```python
from build123d import *

# Parameters (mm, degrees)
SKETCH1_W           = 19.2
SKETCH1_H           = 19.2
SKETCH1_W_2         = 13.2
SKETCH1_H_2         = 13.2
BOSS_EXTRUDE1_DEPTH = 30
CUT_EXTRUDE1_DEPTH  = 30
BOSS_EXTRUDE2_DEPTH = 19.2
SKETCH4_R           = 1.28
CUT_EXTRUDE2_DEPTH  = 30
SKETCH5_R           = 2.18
CUT_EXTRUDE3_DEPTH  = 1
SKETCH6_W           = 10
SKETCH6_H           = 2.5
CUT_EXTRUDE4_DEPTH  = 3
BOSS_EXTRUDE3_DEPTH = 1
SKETCH8_W           = 4
SKETCH8_H           = 3
CUT_EXTRUDE5_DEPTH  = 4
FILLET1_R           = 0.5
FILLET2_R           = 0.5


with BuildPart() as part:
    # Sketch1 → Boss-Extrude1 (new body)
    with BuildSketch(Plane(origin=(0, 0, 0), x_dir=(1, 0, 0), z_dir=(0, 1, 0))):
        Rectangle(SKETCH1_W, SKETCH1_H)
        Rectangle(SKETCH1_W_2, SKETCH1_H_2, mode=Mode.SUBTRACT)
    extrude(amount=-BOSS_EXTRUDE1_DEPTH)

    # Sketch2 → Cut-Extrude1 (cut)
    with BuildSketch(Plane.XY.offset(9.6)):
        Polygon((-9.6, -30), (-9.6, -10), (25.041016151, -30), align=None)
    extrude(amount=-CUT_EXTRUDE1_DEPTH, mode=Mode.SUBTRACT)

    # Sketch3 → Boss-Extrude2 (add)
    with BuildSketch(Plane.XY.offset(9.6)):
        Polygon((-9.6, -10), (-9.6, -12.886751346), (15.662177826, -27.471876514), (15.662177826, -24.585125168), align=None)
    extrude(amount=-BOSS_EXTRUDE2_DEPTH)

    # Sketch4 → Cut-Extrude2 (cut)
    with BuildSketch(Plane(origin=(-6.730127019, -11.656921938, 0), x_dir=(0.866025404, -0.5, 0), z_dir=(0.5, 0.866025404, 0))):
        with Locations(Location((22.558741962, 0, 0), (0, 0, 180))):  # turned: the seam where the file's is
            Circle(SKETCH4_R)
    extrude(amount=-CUT_EXTRUDE2_DEPTH, mode=Mode.SUBTRACT)

    # Sketch5 → Cut-Extrude3 (cut)
    with BuildSketch(Plane(origin=(-6.730127019, -11.656921938, 0), x_dir=(0.866025404, -0.5, 0), z_dir=(0.5, 0.866025404, 0))):
        with Locations(Location((22.558741962, 0, 0), (0, 0, 180))):  # turned: the seam where the file's is
            Circle(SKETCH5_R)
    extrude(amount=-CUT_EXTRUDE3_DEPTH, mode=Mode.SUBTRACT)

    # Sketch6 → Cut-Extrude4 (cut)
    with BuildSketch(Plane(origin=(9.6, 0, 0), x_dir=(0, 0, -1), z_dir=(1, 0, 0))):
        with Locations((0, -15)):
            Rectangle(SKETCH6_W, SKETCH6_H)
    extrude(amount=-CUT_EXTRUDE4_DEPTH, mode=Mode.SUBTRACT)

    # Sketch7 → Boss-Extrude3 (add, symmetric)
    with BuildSketch(Plane.XY):
        Polygon((-6.6, -4.2), (-6.6, -1.2), (-4.6, -1.2), align=None)
        Polygon((6.6, -1.2), (4.6, -1.2), (6.6, -4.2), align=None)
    extrude(amount=BOSS_EXTRUDE3_DEPTH, both=True)

    # Sketch8 → Cut-Extrude5 (cut)
    with BuildSketch(Plane(origin=(0, 0, 0), x_dir=(1, 0, 0), z_dir=(0, 1, 0))):
        with Locations((0, 8.1)):
            Rectangle(SKETCH8_W, SKETCH8_H)
        with Locations((0, -8.1)):
            Rectangle(SKETCH8_W, SKETCH8_H)
    extrude(amount=-CUT_EXTRUDE5_DEPTH, mode=Mode.SUBTRACT)

    # Fillet1
    fillet1_edges = [part.edges().sort_by_distance(p)[0] for p in [
        (-6.6, -1.2, 0),
        (6.6, -1.2, 0),
    ]]
    fillet(fillet1_edges, radius=FILLET1_R)

    # Fillet2
    fillet2_edges = [part.edges().sort_by_distance(p)[0] for p in [
        (-5.8, 0, -9.6),
        (9.6, 0, 0),
        (-5.8, 0, 9.6),
        (5.8, 0, 9.6),
        (5.8, 0, -9.6),
        (-9.6, -6.443375673, 9.6),
        (9.6, -10.542562584, 9.6),
        (9.6, -10.542562584, -9.6),
        (-9.6, -6.443375673, -9.6),
        (9.6, -21.085125168, 0),
        (15.662177826, -24.585125168, 0),
        (12.631088913, -22.835125168, 9.6),
        (15.662177826, -26.028500841, 9.6),
        (12.631088913, -22.835125168, -9.6),
        (15.662177826, -26.028500841, -9.6),
    ]]
    fillet(fillet2_edges, radius=FILLET2_R)


solid = part.part
```
Design review of the part built by this model. Coordinates are the model's own, in mm. A direction names the side the tool comes from. Give positions to 0.01 mm unless a question says otherwise; leave off trailing zeros. Order: outer loops, then holes, each group sorted by start corner. A loop starts at its lowest first (then second) coordinate and runs counter-clockwise, first axis right, second up. Notation, with made-up numbers: (12.25, 0.5) -> (67.25, 0.5) arc R16 ccw to (67.25, 15.5) -> close; hole circle Ø1 at (45, 34). An arc over 180 degrees is marked (long way). Write item = value, one per line. Start each with the question number.
(1) Mouldability with a two-part tool opening along Z and no side actions: class faces 1 (the face through (3, -11, 9.6)), 2 (the face through (-6.6, -6, 0)), 3 (the face through (0, -4, -8)), 4 (the face through (-5, -1.2, 0)) as +Z half, -Z half, draft (parallel to the pull), parting line (faces both ways), or undercut.
(2) We need section D-D on x = 7. Write out the cut boundary in (y, z).
(3) We need section A-A on z = 7.75. Write out the cut boundary in (x, y), plus the area to 3 significant figures.
(4) For faces 5 (the face through (11.07, -23.09, -0.45)), 6 (the face through (2, -2, -8)), 7 (the face through (-6, -2, 1)), list the 3-axis set-ups (+Z, -Z, +X, -X, +Y, -Y) from which the entire face can be reached by the end or side of a thin tool; tool diameter is ignored.
(5) We need section C-C on z = -2.75. Write out the cut boundary in (x, y).
(6) We need section B-B on y = -7. Write out the cut boundary in (x, z), plus the area to 3 significant figures.
(7) To check wall thickness, follow line 1 along X through (y, z) = (-9, 6); line 2 along X through (y, z) = (-7.25, -8.5). State the ranges of each line that lie inside material, in increasing order.
(8) For pin 1 (3.5 mm diameter, centred on y = -4.5, z = 2.5, fed in from +X); pin 2 (4 mm diameter, centred on x = 8.5, z = -6, fed in from -Y); pin 3 (0.9 mm diameter, centred on x = -1, z = -8.5, fed in from +Y), all flat-tipped, find the tip position at first contact; note any pin that passes through.
Numbers:
q1.face_1 = +Z half
q1.face_2 = undercut
q1.face_3 = draft
q1.face_4 = undercut
q2.outline = (-22.47, -9.6) -> (-0.5, -9.6) arc R0.5 ccw to (0, -9.1) -> (0, 9.1) arc R0.5 ccw to (-0.5, 9.6) -> (-22.47, 9.6) -> close; hole (-16.25, -5) -> (-13.75, -5) -> (-13.75, 5) -> (-16.25, 5) -> close
q3.outline = (-9.6, -12.89) -> (15.66, -27.47) -> (15.66, -24.87) arc R0.5 ccw to (15.41, -24.44) -> (9.85, -21.23) arc R0.5 cw to (9.6, -20.8) -> (9.6, -0.5) arc R0.5 ccw to (9.1, 0) -> (2, 0) -> (2, -4) -> (-2, -4) -> (-2, 0) -> (-9.6, 0) -> close
q3.area = 355 mm^2
q4.face_5 = none
q4.face_6 = +Z, -Z, +Y
q4.face_7 = +Y
q5.outline = (-9.6, -12.89) -> (15.66, -27.47) -> (15.66, -24.87) arc R0.5 ccw to (15.41, -24.44) -> (9.85, -21.23) arc R0.5 cw to (9.6, -20.8) -> (9.6, -16.25) -> (6.6, -16.25) -> (6.6, -19.35) -> (-6.6, -11.73) -> (-6.6, 0) -> (-9.6, 0) -> close; (6.6, -13.75) -> (9.6, -13.75) -> (9.6, -0.5) arc R0.5 ccw to (9.1, 0) -> (6.6, 0) -> close
q6.outline = (-9.6, -9.1) arc R0.5 ccw to (-9.1, -9.6) -> (9.1, -9.6) arc R0.5 ccw to (9.6, -9.1) -> (9.6, 9.1) arc R0.5 ccw to (9.1, 9.6) -> (-9.1, 9.6) arc R0.5 ccw to (-9.6, 9.1) -> close; hole (-6.6, -6.6) -> (6.6, -6.6) -> (6.6, 6.6) -> (-6.6, 6.6) -> close
q6.area = 194 mm^2
q7.line_1 = -9.6 to -6.6, 6.6 to 9.6
q7.line_2 = -9.6 to 9.6
q8.pin_1 = 9.6
q8.pin_2 = -24.49
q8.pin_3 = -4
